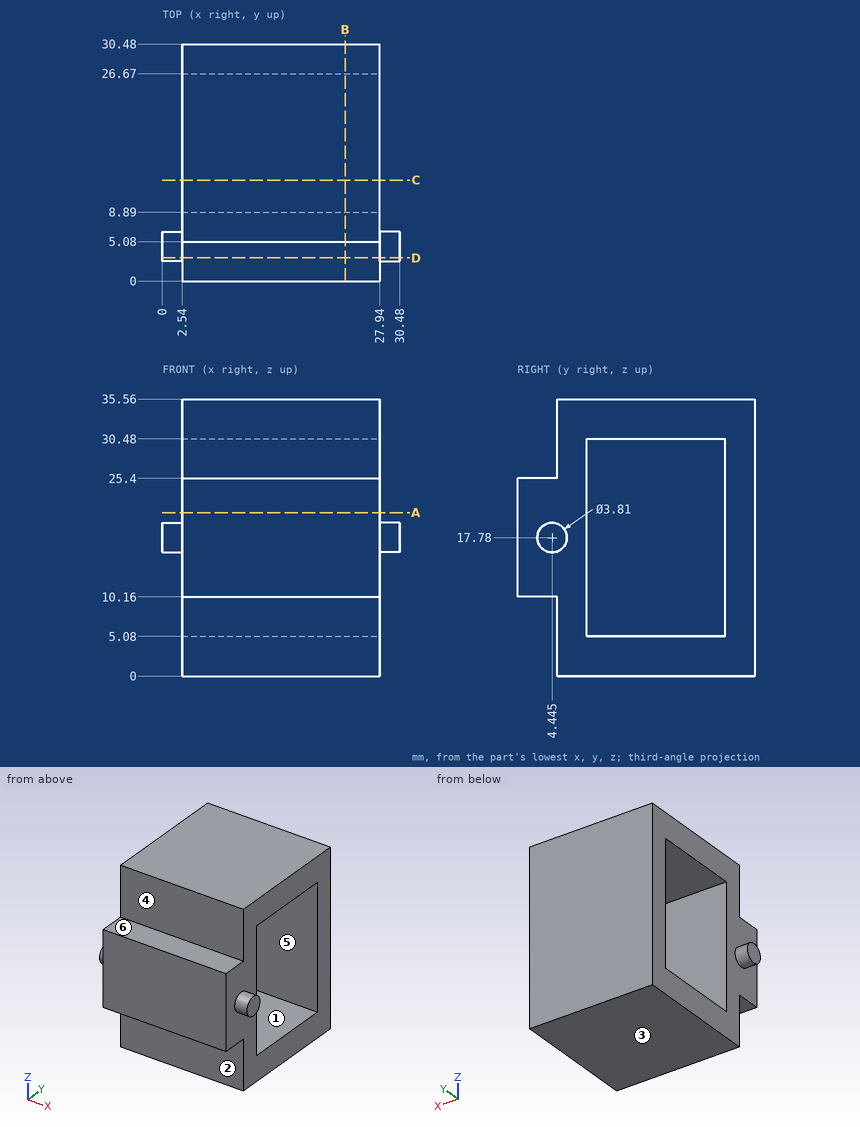
Geometry: see drawing. Coordinates: mm, zero at the bounding-box minimum. A direction names the side the tool comes from. Coordinates: 2 decimals unless noted, no trailing zeros. Loops run counter-clockwise (first coordinate to the right, second up) from the corner with the lowest first, then second, coordinate; pieces in that order, holes last.
(1) Section B-B on x = 23.5. Return the cut outline in (y, z), then the cut area to 3 significant figures.
(2) Section A-A on z = 21. Return the cut outline in (x, y), then the cut area to 3 significant figures.
(3) Section D-D on y = 3. Return the cut outline in (x, z).
(4) Section C-C on y = 13. Return the cut outline in (x, z), then the cut area to 3 significant figures.
(5) Pull-direction query (Y, two-part tool) for the marked faces 4, 5 and 6; classes: released by +Y, released by -Y, zero draft, split by the parting line, or undercut.
(6) Material intervals for probe 1 along Z at (x, y) = (12, 11); probe 2 along Y at (x, z) = (25, 7.5); probe 3 along Y at (x, z) = (25, 13), sorted ascending.
(7) First-contact query: pin 1 Ø3 at (x, z) = (19, 7.5) entering from -Y; pin 2 Ø2 at (x, z) = (21.5, 18.5) entering from -Y; pin 3 Ø1.5 at (x, y) = (21, 2.5) entering from +Z; pin 4 Ø6 at (y, z) = (23, 10.5) entering from -X. Flat tips, straight axial feed; report the tip coordinate or a pass-through.
(8) Set-up query: the marked faces 1, 2 and 3. Return all of +Z, -Z, +X, -X, +Y, -Y with unobstructed straight access to the full face (end or side cutting, diameter ignored); none if empty.
Data:
1. outline: (0, 10.16) - (5.08, 10.16) - (5.08, 0) - (30.48, 0) - (30.48, 35.56) - (5.08, 35.56) - (5.08, 25.4) - (0, 25.4) - close; hole (8.89, 5.08) - (26.67, 5.08) - (26.67, 30.48) - (8.89, 30.48) - close
1. area: 529 mm2
2. outline: (2.54, 0) - (27.94, 0) - (27.94, 8.89) - (2.54, 8.89) - close; (2.54, 26.67) - (27.94, 26.67) - (27.94, 30.48) - (2.54, 30.48) - close
2. area: 323 mm2
3. outline: (0, 16.54) - (2.54, 16.54) - (2.54, 10.16) - (27.94, 10.16) - (27.94, 16.54) - (30.48, 16.54) - (30.48, 19.02) - (27.94, 19.02) - (27.94, 25.4) - (2.54, 25.4) - (2.54, 19.02) - (0, 19.02) - close
4. outline: (2.54, 0) - (27.94, 0) - (27.94, 5.08) - (2.54, 5.08) - close; (2.54, 30.48) - (27.94, 30.48) - (27.94, 35.56) - (2.54, 35.56) - close
4. area: 258 mm2
5. face 4: released by -Y
5. face 5: undercut
5. face 6: zero draft
6. probe 1: z = 0 to 5.08, 30.48 to 35.56
6. probe 2: y = 5.08 to 8.89, 26.67 to 30.48
6. probe 3: y = 0 to 8.89, 26.67 to 30.48
7. pin 1: stops at y = 5.08
7. pin 2: stops at y = 0
7. pin 3: stops at z = 25.4
7. pin 4: passes through
8. face 1: +X, -X
8. face 2: -Z, +X, -X, -Y
8. face 3: -Z, +X, -X, +Y, -Y
